from build123d import *

# Parameters (mm, degrees)
SKETCH1_R               = 78.35
SKETCH1_R_2             = 76.35
BOSS_EXTRUDE1_DEPTH     = 1700
SKETCH5_R               = 15
CUT_EXTRUDE2_DEPTH      = 1704.607186237
SKETCH6_W               = 4.8
SKETCH6_H               = 270
CUT_EXTRUDE3_DEPTH      = 1704.607186346
CIRPATTERN1_COUNT       = 2
CIRPATTERN1_ANGLE       = 90
CUT_EXTRUDE4_DEPTH      = 17.5
CUT_EXTRUDE4_DEPTH_BACK = 17.5


with BuildPart() as part:
    # Sketch1 → Boss-Extrude1 (new body)
    with BuildSketch(Plane.XY):
        Circle(SKETCH1_R)
        Circle(SKETCH1_R_2, mode=Mode.SUBTRACT)
    extrude(amount=BOSS_EXTRUDE1_DEPTH)

    # Sketch5 → Cut-Extrude2 (cut, through all)
    with BuildSketch(Plane(origin=(0, 0, 0), x_dir=(0, 0, -1), z_dir=(0.7071067811865489, -0.7071067811865462, 0))):
        with Locations(Location((-1034.89, 0, 0), (0, 0, 270))):
            Circle(SKETCH5_R)
    extrude(amount=CUT_EXTRUDE2_DEPTH, mode=Mode.SUBTRACT)

    # Sketch6 → Cut-Extrude3 (cut, symmetric)
    with BuildSketch(Plane(origin=(0, 0, 0), x_dir=(1, 0, 0), z_dir=(0, 1, 0))):
        with Locations((0, -150)):
            Rectangle(SKETCH6_W, SKETCH6_H)
    cut_extrude3 = extrude(amount=CUT_EXTRUDE3_DEPTH, both=True, mode=Mode.SUBTRACT)

    # CirPattern1: Cut-Extrude3 ×2 about axis
    cirpattern1_axis = Axis((0, 0, 0), (0, 0, 1))
    for i in range(1, CIRPATTERN1_COUNT):
        add(cut_extrude3.rotate(cirpattern1_axis, i * CIRPATTERN1_ANGLE / (CIRPATTERN1_COUNT - 1)), mode=Mode.SUBTRACT)

    # Sketch7 → Cut-Extrude4 (cut, two sides: drawn at the far end of the back side and taken through both)
    with BuildSketch(Plane.XY.offset(1035).offset(-CUT_EXTRUDE4_DEPTH_BACK)):
        with BuildLine():
            Line((65.460051126, -39.297636146), (67.174787239, -40.327043772))
            ThreePointArc((67.174787239, -40.327043772), (67.934531185, -39.03360056), (68.669373093, -37.725849215))
            Line((68.669373093, -37.725849215), (66.916485458, -36.762840939))
            ThreePointArc((66.916485458, -36.762840939), (66.20040148, -38.03720999), (65.460051126, -39.297636146))
        make_face()
        with BuildLine():
            Line((37, -66.785645913), (37.969220694, -68.535106186))
            ThreePointArc((37.969220694, -68.535106186), (39.274356912, -67.795629573), (40.565096747, -67.031301837))
            Line((40.565096747, -67.031301837), (39.529612465, -65.320228401))
            ThreePointArc((39.529612465, -65.320228401), (38.271820679, -66.065045538), (37, -66.785645913))
        make_face()
        with BuildLine():
            Line((39.529612465, -65.320228401), (40.565096747, -67.031301837))
            ThreePointArc((40.565096747, -67.031301837), (48.389164921, -61.621515871), (55.5, -55.303458301))
            Line((55.5, -55.303458301), (54.083280153, -53.891755472))
            ThreePointArc((54.083280153, -53.891755472), (47.15395969, -60.048535249), (39.529612465, -65.320228401))
        make_face()
        with BuildLine():
            Line((54.083280153, -53.891755472), (55.5, -55.303458301))
            ThreePointArc((55.5, -55.303458301), (61.792791684, -48.170254265), (67.174787239, -40.327043772))
            Line((67.174787239, -40.327043772), (65.460051126, -39.297636146))
            ThreePointArc((65.460051126, -39.297636146), (60.215438992, -46.940637053), (54.083280153, -53.891755472))
        make_face()
    extrude(amount=CUT_EXTRUDE4_DEPTH + CUT_EXTRUDE4_DEPTH_BACK, mode=Mode.SUBTRACT)


solid = part.part
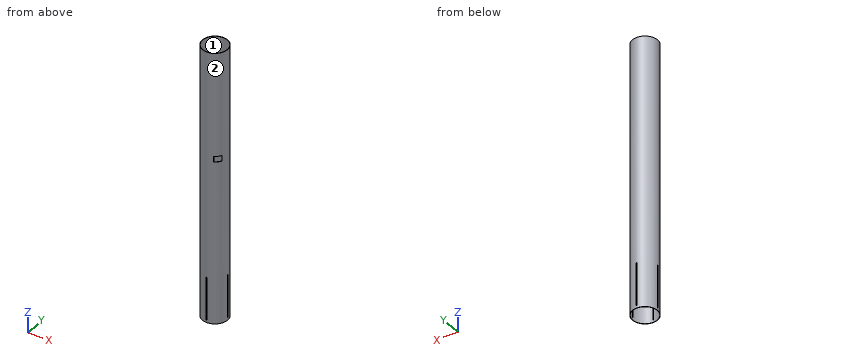
Design review of the part built by this model. Coordinates are the model's own, in mm. Face numbers are marked on the shaded views. Coordinates: 2 decimals unless noted, no trailing zeros. Loops run counter-clockwise (first coordinate to the right, second up) from the corner with the lowest first, then second, coordinate; pieces in that order, holes last. Notation, with made-up numbers: (41, -12) - (82, -12) arc R18 ccw to (82, 11) - close; hole circle Ø9 at (-10, -19.5). An arc over 180 degrees is marked (long way). Use CSV: the item, a comma, the result in double quotes. Start each with the question number.
1. Mouldability with a two-part tool opening along X and no side actions: class the marked faces 1 and 2 as released by +X, released by -X, zero draft, split by the parting line, or undercut.
2. To check wall thickness, follow probe 1 along X at (y, z) = (0, 696.5); probe 2 along Y at (x, z) = (-6.5, 940). State the ranges of each line that lie inside material, in increasing order.
3. Add section C-C on z = 901. Give the boundary of the cut face in (x, y), plus the area to 3 significant figures.
4. Clearance check with flat-ended pins moving along their axes: pin 1 (1.5 mm diameter, centred on x = 1, z = 718, fed in from -Y); pin 2 (6 mm diameter, centred on y = 18, z = 520, fed in from +X); pin 3 (4 mm diameter, centred on x = -53, z = 659.5, fed in from -Y); pin 4 (1 mm diameter, centred on x = 0.5, y = -77.5, fed in from -Z). State where each tip first meets the part, or that it passes through.
5. Add section B-B on x = -20.5. Give the boundary of the cut face in (y, z), plus the area to 3 significant figures.
Resolved:
1,face 1,"undercut"
1,face 2,"split by the parting line"
2,probe 1,"-78.35 to -76.35, 76.35 to 78.35"
2,probe 2,"-78.08 to -76.07, 76.07 to 78.08"
3,outline,"circle Ø156.7 at (0, 0); hole circle Ø152.7 at (0, 0)"
3,area,"972 mm2"
4,pin 1,"y = -78.35"
4,pin 2,"x = 76.9"
4,pin 3,"y = -59.48"
4,pin 4,"z = 0"
5,outline,"(-75.62, 0) - (-73.55, 0) - (-73.55, 1700) - (-75.62, 1700) - close; (73.55, 0) - (75.62, 0) - (75.62, 1700) - (73.55, 1700) - close"
5,area,"7,050 mm2"
